Here's how the part is built. I have some questions about the finished solid (model axes, mm). Face numbers are marked on the shaded views. A direction names the side the tool comes from. Round coordinates to 2 decimals unless told otherwise and drop trailing zeros. Write each loop counter-clockwise with the first axis right and the second up, starting at its lowest first coordinate (ties: lowest second). Pieces come first, ordered by that corner, then holes. Notation, with made-up numbers: (36, 81.5) -> (56, 81.5) arc R28 ccw to (56, 106.5) -> close; hole circle Ø9 at (-39, -4). An arc over 180 degrees is marked (long way). Answer in a Markdown table with one row per item. Add a question column.
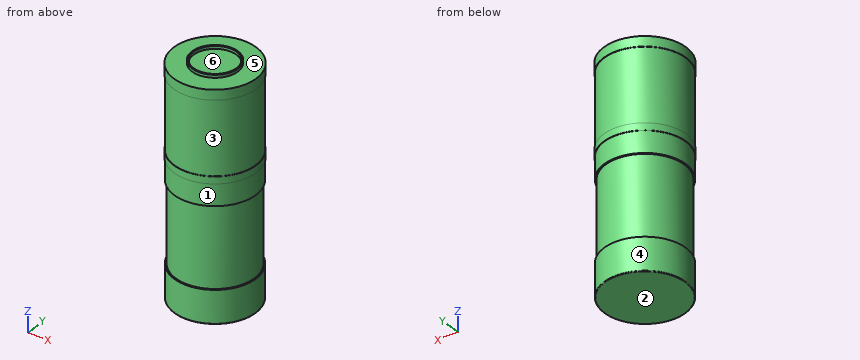
from build123d import *

# Parameters (mm, degrees)
ESQUISSE1_R        = 28.5
BOSS_EXTRU_1_DEPTH = 23
ESQUISSE3_R        = 27.5
BOSS_EXTRU_2_DEPTH = 56
ESQUISSE4_R        = 28.5
BOSS_EXTRU_3_DEPTH = 15
ESQUISSE5_R        = 28.75
BOSS_EXTRU_4_DEPTH = 5
ESQUISSE6_R        = 28.5
BOSS_EXTRU_5_DEPTH = 51
ESQUISSE7_R        = 28.75
BOSS_EXTRU_6_DEPTH = 7
CONG_1_R           = 0.5
ESQUISSE8_R        = 16
ESQUISSE8_R_2      = 15
BOSS_EXTRU_7_DEPTH = 2


with BuildPart() as part:
    # Esquisse1 → Boss.-Extru.1 (new body)
    with BuildSketch(Plane.XY):
        Circle(ESQUISSE1_R)
    extrude(amount=BOSS_EXTRU_1_DEPTH)

    # Esquisse3 → Boss.-Extru.2 (add)
    with BuildSketch(Plane.XY.offset(23)):
        Circle(ESQUISSE3_R)
    extrude(amount=BOSS_EXTRU_2_DEPTH)

    # Esquisse4 → Boss.-Extru.3 (add)
    with BuildSketch(Plane.XY.offset(79)):
        Circle(ESQUISSE4_R)
    extrude(amount=BOSS_EXTRU_3_DEPTH)

    # Esquisse5 → Boss.-Extru.4 (add)
    with BuildSketch(Plane.XY.offset(94)):
        Circle(ESQUISSE5_R)
    extrude(amount=BOSS_EXTRU_4_DEPTH)

    # Esquisse6 → Boss.-Extru.5 (add)
    with BuildSketch(Plane.XY.offset(99)):
        Circle(ESQUISSE6_R)
    extrude(amount=BOSS_EXTRU_5_DEPTH)

    # Esquisse7 → Boss.-Extru.6 (add)
    with BuildSketch(Plane.XY.offset(150)):
        Circle(ESQUISSE7_R)
    extrude(amount=BOSS_EXTRU_6_DEPTH)

    # Congé1
    cong_1_edges = [part.edges().sort_by_distance(p)[0] for p in [
        (-28.5, 0, 0),
    ]]
    fillet(cong_1_edges, radius=CONG_1_R)

    # Esquisse8 → Boss.-Extru.7 (add)
    with BuildSketch(Plane.XY.offset(157)):
        Circle(ESQUISSE8_R)
        Circle(ESQUISSE8_R_2, mode=Mode.SUBTRACT)
    extrude(amount=BOSS_EXTRU_7_DEPTH)


solid = part.part
Item 1: If we section it at D-D on z = 117: Please give me the cut outline in (x, y).
Item 2: If we section it at C-C on z = 70: Please give me the cut outline in (x, y), then the cut area to 3 significant figures.
Item 3: For P1, Ø8, axis at x = 3, y = -3, coming from the +Z side; P2, Ø3, axis at y = -17, z = 133.5, coming from the -X side; P3, Ø3, axis at y = -14.5, z = 22, coming from the -X side, each with a flat end and sliding along its axis, tell me the tip position at first contact or that it passes through.
Item 4: If we mould it in two halves opening along X, with no side actions, what happens to the marked faces 4, 5 and 6? For each: pulls with the +X half, pulls with the -X half, needs draft (parallel to the pull), parting line crosses it, or undercut.
Item 5: On a 3-axis mill with a long thin cutter (end or side, diameter ignored), from which of +Z, -Z, +X, -X, +Y, -Y can I reach the whole of each face in a straight line? I mean the marked faces 1, 2 and 3. Say none if no direction works.
Item 6: I need wall thicknesses on line 1 along Y through (x, z) = (0, 158.05); line 2 along Z through (x, y) = (1, -18.5); line 3 along Z through (x, y) = (13.5, 25). Which ranges of each line are inside material? Lowest first, please. Write a range as from..to.
Results list:
| question | item | result |
|---|---|---|
| 1 | outline | circle Ø57 at (0, 0) |
| 2 | outline | circle Ø55 at (0, 0) |
| 2 | area | 2,380 mm² |
| 3 | P1 | z = 157 |
| 3 | P2 | x = -23.92 |
| 3 | P3 | x = -25.36 |
| 4 | face 4 | parting line crosses it |
| 4 | face 5 | needs draft |
| 4 | face 6 | undercut |
| 5 | face 1 | -Z |
| 5 | face 2 | -Z, +X, -X, +Y, -Y |
| 5 | face 3 | none |
| 6 | line 1 | -16..-15, 15..16 |
| 6 | line 2 | 0..157 |
| 6 | line 3 | 0.22..23, 79..157 |
